```python
from build123d import *

# Parameters (mm, degrees)
F1_DEPTH = 50
F3_DEPTH = 31
F4_R     = 26
F5_DEPTH = 15


with BuildPart() as f1:
    # F0 (on Front) → F1 (new body)
    with BuildSketch(Plane.XZ):
        with BuildLine():
            ThreePointArc((55.5, 51.9206124771), (30.2492433933, 69.7207521053), (0, 76))
            ThreePointArc((0, 76), (-76, 0), (0, -76))
            ThreePointArc((0, -76), (30.2492433933, -69.7207521053), (55.5, -51.9206124771))
            ThreePointArc((55.5, -51.9206124771), (35, 0), (55.5, 51.9206124771))
        make_face()
        with BuildLine():
            Line((111, 76), (0, 76))
            ThreePointArc((0, 76), (30.2492433933, 69.7207521053), (55.5, 51.9206124771))
            ThreePointArc((55.5, 51.9206124771), (80.7507566067, 69.7207521053), (111, 76))
        make_face()
        with BuildLine():
            ThreePointArc((55.5, -51.9206124771), (30.2492433933, -69.7207521053), (0, -76))
            Line((0, -76), (111, -76))
            ThreePointArc((111, -76), (80.7507566067, -69.7207521053), (55.5, -51.9206124771))
        make_face()
        with BuildLine():
            ThreePointArc((111, 76), (80.7507566067, 69.7207521053), (55.5, 51.9206124771))
            ThreePointArc((55.5, 51.9206124771), (70.6894617323, 27.9105714739), (76, 0))
            ThreePointArc((76, 0), (70.6894617323, -27.9105714739), (55.5, -51.9206124771))
            ThreePointArc((55.5, -51.9206124771), (80.7507566067, -69.7207521053), (111, -76))
            ThreePointArc((111, -76), (164.7401153702, -53.7401153702), (187, 0))
            ThreePointArc((187, 0), (164.7401153702, 53.7401153702), (111, 76))
        make_face()
        with BuildLine():
            ThreePointArc((76, 0), (70.6894617323, 27.9105714739), (55.5, 51.9206124771))
            ThreePointArc((55.5, 51.9206124771), (35, 0), (55.5, -51.9206124771))
            ThreePointArc((55.5, -51.9206124771), (70.6894617323, -27.9105714739), (76, 0))
        make_face()
    extrude(amount=F1_DEPTH)

    # F2 (on face) → F3 (cut)
    with BuildSketch(Plane.XZ.offset(50)):
        with BuildLine():
            ThreePointArc((55.5, 31.870833061), (32.0645184285, 55.3883260078), (0, 64))
            ThreePointArc((0, 64), (-64, 0), (0, -64))
            ThreePointArc((0, -64), (32.0645184285, -55.3883260078), (55.5, -31.870833061))
            ThreePointArc((55.5, -31.870833061), (47, 0), (55.5, 31.870833061))
        make_face()
        with BuildLine():
            Line((111, 64), (0, 64))
            ThreePointArc((0, 64), (32.0645184285, 55.3883260078), (55.5, 31.870833061))
            ThreePointArc((55.5, 31.870833061), (78.9354815715, 55.3883260078), (111, 64))
        make_face()
        with BuildLine():
            ThreePointArc((55.5, -31.870833061), (32.0645184285, -55.3883260078), (0, -64))
            Line((0, -64), (111, -64))
            ThreePointArc((111, -64), (78.9354815715, -55.3883260078), (55.5, -31.870833061))
        make_face()
        with BuildLine():
            ThreePointArc((111, 64), (78.9354815715, 55.3883260078), (55.5, 31.870833061))
            ThreePointArc((55.5, 31.870833061), (61.838499335, 16.4924225025), (64, 0))
            ThreePointArc((64, 0), (61.838499335, -16.4924225025), (55.5, -31.870833061))
            ThreePointArc((55.5, -31.870833061), (78.9354815715, -55.3883260078), (111, -64))
            ThreePointArc((111, -64), (156.2548339959, -45.2548339959), (175, 0))
            ThreePointArc((175, 0), (156.2548339959, 45.2548339959), (111, 64))
        make_face()
        with BuildLine():
            ThreePointArc((64, 0), (61.838499335, 16.4924225025), (55.5, 31.870833061))
            ThreePointArc((55.5, 31.870833061), (47, 0), (55.5, -31.870833061))
            ThreePointArc((55.5, -31.870833061), (61.838499335, -16.4924225025), (64, 0))
        make_face()
    extrude(amount=-F3_DEPTH, mode=Mode.SUBTRACT)

    # F4 (on face) → F5 (cut)
    with BuildSketch(Plane.XZ.offset(19)):
        with Locations((10.5443401262, 0)):
            Circle(F4_R)
    extrude(amount=-F5_DEPTH, mode=Mode.SUBTRACT)

    # F7 (on offset) → F8 (revolve, cut)
    with BuildSketch(Plane.YZ.offset(111)):
        Polygon((0, 0), (0, 11), (-2, 11), (-2, 18.5), (-7, 18.5), (-7, 23.5), (-19, 23.5), (-19, 0), align=None)
    revolve(axis=Axis((111, -17.0189570636, 0), (0, 1, 0)), mode=Mode.SUBTRACT)


solid = f1.part
```
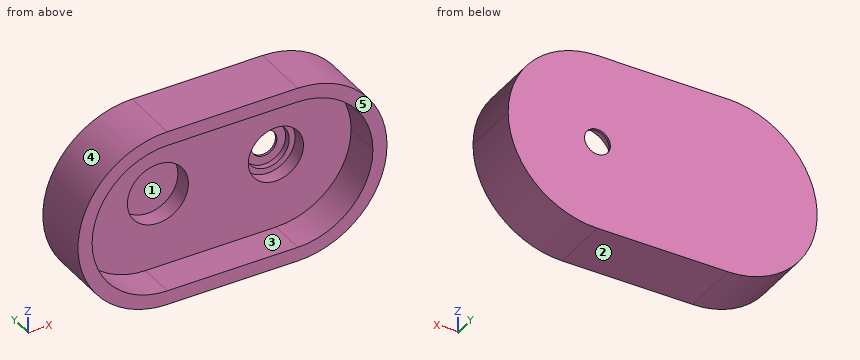
Model file for the job. Use its own axes, mm. Face numbers are marked on the shaded views. A direction names the side the tool comes from. Round coordinates to 2 decimals unless told otherwise and drop trailing zeros. Write each loop counter-clockwise with the first axis right and the second up, starting at its lowest first coordinate (ties: lowest second). Pieces come first, ordered by that corner, then holes. Notation, with made-up numbers: (-5.5, 63) -> (3.5, 63) arc R29 cw to (3.5, 98) -> close; hole circle Ø6 at (80, 30). An arc over 180 degrees is marked (long way). Answer as CSV lines item,"result".
1. Slice it at B-B, the plane y = -36. List the corners of the cut face in (x, z).
Resolved:
outline,"(0, -76) -> (111, -76) arc R76 ccw to (111, 76) -> (0, 76) arc R76 ccw to start; hole (0, -64) -> (111, -64) arc R64 ccw to (111, 64) -> (0, 64) arc R64 ccw to start"
2. Slice it at C-C, the plane z = -59. List the corners of the cut face in (x, y), plus the area to 3 significant figures.
Resolved:
outline,"(-47.91, -50) -> (-24.8, -50) -> (-24.8, -19) -> (135.8, -19) -> (135.8, -50) -> (158.91, -50) -> (158.91, 0) -> (-47.91, 0) -> close"
area,"5,360 mm²"
3. Slice it at D-D, the plane x = 13. List the corners of the cut face in (y, z), plus the area to 3 significant figures.
Resolved:
outline,"(-50, -76) -> (0, -76) -> (0, 76) -> (-50, 76) -> (-50, 64) -> (-19, 64) -> (-19, 25.88) -> (-4, 25.88) -> (-4, -25.88) -> (-19, -25.88) -> (-19, -64) -> (-50, -64) -> close"
area,"2,860 mm²"
4. Mould opens along X. For the marked faces 3, 4 and 5 say: +X half, -X half, draft (parallel to the pull), parting line (faces both ways), or undercut.
Resolved:
face 3,"undercut"
face 4,"-X half"
face 5,"draft"
5. Slice it at A-A, the plane x = 68. List the corners of the cut face in (y, z).
Resolved:
outline,"(-50, -76) -> (0, -76) -> (0, 76) -> (-50, 76) -> (-50, 64) -> (-19, 64) -> (-19, -64) -> (-50, -64) -> close"
6. Pin check, flat tips, straight feed: pin 1 Ø4 at (y, z) = (-39, -21) entering from -X; pin 2 Ø12 at (x, y) = (146, -24) entering from -Z; pin 3 Ø4 at (x, y) = (145.5, -9) entering from -Z. Stop position of each tip, or through.
Resolved:
pin 1,"x = -73.59"
pin 2,"z = -70.25"
pin 3,"z = -68.7"
7. Tool access for the marked faces 1 and 2: list every direction of +Z, -Z, +X, -X, +Y, -Y with a clear straight run to the whole face (end or side of a thin tool).
Resolved:
face 1,"-Y"
face 2,"-Z, +X, -X, +Y, -Y"
8. Drill centre lines: line 1 (X direction, y = -14.5, z = 6.5); line 2 (X direction, y = -3.3, z = 0); line 3 (X direction, y = -7.5, z = 9). Where is each one in solid material? Low to high.
Resolved:
line 1,"-75.72 to -14.63, 35.72 to 88.42, 133.58 to 186.72"
line 2,"-76 to 92.5, 129.5 to 187"
line 3,"-75.47 to -13.85, 34.94 to 89.29, 132.71 to 186.47"
